```python
from build123d import *

# Parameters (mm, degrees)
F0_W     = 25
F0_H     = 18
F1_DEPTH = 8
F3_DEPTH = 25
F4_R     = 2.075
F5_R     = 2.075
F6_DEPTH = 25
F7_R     = 1
F8_R     = 0.5


with BuildPart() as f1:
    # F0 (on Top) → F1 (new body)
    with BuildSketch(Plane.XY):
        Rectangle(F0_W, F0_H)
    extrude(amount=F1_DEPTH)

    # F2 (on face) → F3 (cut)
    with BuildSketch(Plane.XZ.offset(9)):
        with BuildLine():
            Line((4.8989794856, 8), (-4.8989794856, 8))
            ThreePointArc((-4.8989794856, 8), (0, 4), (4.8989794856, 8))
        make_face()
    extrude(amount=-F3_DEPTH, mode=Mode.SUBTRACT)

    # F4 (on face) + F5 (on face) → F6 (cut)
    with BuildSketch(Plane.XY.offset(8)):
        with Locations((-8.6994897428, 0)):
            Circle(F4_R)
    with BuildSketch(Plane.XY.offset(8)):
        with Locations((8.6994897428, 0)):
            Circle(F5_R)
    extrude(amount=-F6_DEPTH, mode=Mode.SUBTRACT)

    # F7
    f7_edges = [f1.edges().sort_by_distance(p)[0] for p in [
        (-12.5, -9, 4),
        (12.5, -9, 4),
        (12.5, 9, 4),
        (-12.5, 9, 4),
    ]]
    fillet(f7_edges, radius=F7_R)

    # F8
    f8_edges = [f1.edges().sort_by_distance(p)[0] for p in [
        (-12.5, 0, 0),
    ]]
    fillet(f8_edges, radius=F8_R)


solid = f1.part
```
Input: part model. Units: mm. Frame: model coordinates. Round coordinates to 2 decimals unless told otherwise and drop trailing zeros. Order: outer loops, then holes, each group sorted by start corner. A loop starts at its lowest first (then second) coordinate and runs counter-clockwise, first axis right, second up. Notation, with made-up numbers: (52.25, 30.5) - (68.25, 30.5) arc R22 cw to (68.25, 57.5) - close; hole circle Ø10 at (-16, 38). An arc over 180 degrees is marked (long way). One line per question, with ' | ' between items. Start each with the question number.
1) Pull-direction query (Y, two-part tool) for faces 1 (the cylindrical face through (12.199, 8.715, 4.302)), 2 (the cylindrical face through (-6.72, 0.62, 4.06)), 3 (the flat face through (-10, 2, 8)); classes: +Y half, -Y half, draft (parallel to the pull), parting line (faces both ways), or undercut.
2) Cut plane C-C, the plane x = 4. Return the cut outline in (y, z).
3) Cut plane B-B, the plane z = 2. Return the cut outline in (x, y) (3 decimals), then the cut area to 3 significant figures.
4) Contact query for a flat-ended pin moving along its axis: P1, Ø2.5, axis at x = -8.7, y = 0, coming from the -Z side. Output: stop coordinate, or through.
5) Cut plane D-D, the plane y = 2.5. Return the cut outline in (x, z), then the cut area to 3 significant figures.
6) Cut plane A-A, the plane y = 0. Return the cut outline in (x, z).
7) Ray query, probe 1 along X at (y, z) = (0.25, 1.5); probe 2 along Y at (x, z) = (-7.5, 6.25); probe 3 along Y at (x, z) = (7, 7.5). Return the intervals inside material, ascending.
Worked out:
1) face 1: +Y half | face 2: undercut | face 3: draft
2) outline: (-9, 0.5) arc R0.5 ccw to (-8.5, 0) - (8.5, 0) arc R0.5 ccw to (9, 0.5) - (9, 6) - (-9, 6) - close
3) outline: (-12.5, -8) arc R1 ccw to (-11.5, -9) - (11.5, -9) arc R1 ccw to (12.5, -8) - (12.5, 8) arc R1 ccw to (11.5, 9) - (-11.5, 9) arc R1 ccw to (-12.5, 8) - close; hole circle Ø4.15 at (-8.699, 0); hole circle Ø4.15 at (8.699, 0) | area: 422 mm^2
4) P1: passes through
5) outline: (-12.5, 0.5) arc R0.5 ccw to (-12, 0) - (12, 0) arc R0.5 ccw to (12.5, 0.5) - (12.5, 8) - (4.9, 8) arc R5 cw to (-4.9, 8) - (-12.5, 8) - close | area: 171 mm^2
6) outline: (-12.5, 0.5) arc R0.5 ccw to (-12, 0) - (-10.77, 0) - (-10.77, 8) - (-12.5, 8) - close; (-6.62, 0) - (6.62, 0) - (6.62, 8) - (4.9, 8) arc R5 cw to (-4.9, 8) - (-6.62, 8) - close; (10.77, 0) - (12, 0) arc R0.5 ccw to (12.5, 0.5) - (12.5, 8) - (10.77, 8) - close
7) probe 1: x = -12.5 to -10.76, -6.64 to 6.64, 10.76 to 12.5 | probe 2: y = -9 to -1.69, 1.69 to 9 | probe 3: y = -9 to -1.19, 1.19 to 9
